Design review of the part built by this model. Coordinates are the model's own, in mm. A direction names the side the tool comes from. Coordinates: 2 decimals unless noted, no trailing zeros. Write each loop counter-clockwise with the first axis right and the second up, starting at its lowest first coordinate (ties: lowest second). Pieces come first, ordered by that corner, then holes. Notation, with made-up numbers: (87, -10.75) - (139, -10.75) arc R28 cw to (139, 19.25) - close; hole circle Ø10 at (-2, 57.25). An arc over 180 degrees is marked (long way). Answer as CSV lines item,"result". Start each with the question number.
Q1. Machinability: for faces 1 (the face through (-11, 10, 6)), 2 (the face through (-23.846, 4.93, -7.509)), which of the approach directions +Z, -Z, +X, -X, +Y, -Y give a long, thin tool a straight path to every point of the face, cutting with its end or side? Answer none if there is none.
Q2. We need section B-B (z = 0). Write out the cut boundary in (x, y), plus the area to 3 significant figures.
Q3. We need section D-D (z = 20). Write out the cut boundary in (x, y), plus the area to 3 significant figures.
Q4. We need section A-A (x = 20). Write out the cut boundary in (y, z), plus the area to 3 significant figures.
Q5. Mouldability with a two-part tool opening along X and no side actions: class faces 3 (the face through (0, 110, 11)), 4 (the face through (-17, 5, 0)), 5 (the face through (-3.2, 59.3, 10)), 6 (the face through (-11.99, 59.3, 0.53)) as pulls with the +X half, pulls with the -X half, needs draft (parallel to the pull), parting line crosses it, or undercut.
Q6. We need section C-C (x = 0). Write out the cut boundary in (y, z).
Q7. For line 1 along Y through (x, z) = (9, 1.5); line 2 along Z through (x, y) = (2.5, 32.5); line 3 along X through (y, z) = (43, 0), list the stretches that pass through material, from the lowest coordinate up. Write a range as [from, to].
Q8. Clearance check with flat-ended pins moving along their axes: pin 1 (10.5 mm diameter, centred on x = 2.5, z = -2, fed in from +Y); pin 2 (5.5 mm diameter, centred on x = -20, z = 0, fed in from +Y); pin 3 (1 mm diameter, centred on y = 21.5, z = 8.5, fed in from +X); pin 4 (5 mm diameter, centred on x = -2.5, y = 76.5, fed in from +Z). State where each tip first meets the part, or that it passes through.
Autodesk Inventor part; units mm, degrees
ref_plane "YZ Plane" through (0, 0, 0) normal (1, 0, 0) x (0, 1, 0)
ref_plane "XZ Plane" through (0, 0, 0) normal (0, 1, 0) x (-1, 0, 0)
ref_plane "XY Plane" through (0, 0, 0) normal (0, 0, 1) x (1, 0, 0)
sketch "Boceto1" plane through (0, 0, 0) normal (0, 1, 0) x (-1, 0, 0)
  circle A0 centre (0, 0) radius 25
  circle A1 centre (20, 0) radius 3
  circle A2 centre (0, 20) radius 3
  circle A3 centre (-20, 0) radius 3
  circle A4 centre (0, -20) radius 3
  dimension "d0" = 50
  dimension "d2" = 6
  dimension "d5" = 360
extrude "Extrusión1" add sketch "Boceto1" along normal blind 10
sketch "Boceto2" plane through (0, 10, 0) normal (0, 1, 0) x (1, 0, 0)
  circle A0 centre (0, 0) radius 12
  circle A1 centre (0, 0) radius 10.5
  dimension "d9" = 24
  dimension "d10" = 21
extrude "Extrusión2" add sketch "Boceto2" along normal blind 100 contours A0 | A1
sketch "Boceto3" plane through (0, 110, 0) normal (0, 1, 0) x (1, 0, 0)
  circle A0 centre (0, 0) radius 12
hole "Agujero1" at (0, 110, 0) direction (0, -1, 0) diameter 21 depth 100
Results list:
1,face 1,"+Y"
1,face 2,"+Y, -Y"
2,outline,"(-25, 0) - (-23, 0) - (-23, 10) - (-25, 10) - close; (-17, 0) - (17, 0) - (17, 10) - (12, 10) - (12, 110) - (10.5, 110) - (10.5, 10) - (-10.5, 10) - (-10.5, 110) - (-12, 110) - (-12, 10) - (-17, 10) - close; (23, 0) - (25, 0) - (25, 10) - (23, 10) - close"
2,area,"680 mm2"
3,outline,"(-15, 0) - (-3, 0) - (-3, 10) - (-15, 10) - close; (3, 0) - (15, 0) - (15, 10) - (3, 10) - close"
3,area,"240 mm2"
4,outline,"(0, -15) - (10, -15) - (10, -3) - (0, -3) - close; (0, 3) - (10, 3) - (10, 15) - (0, 15) - close"
4,area,"240 mm2"
5,face 3,"needs draft"
5,face 4,"undercut"
5,face 5,"undercut"
5,face 6,"parting line crosses it"
6,outline,"(0, -25) - (10, -25) - (10, -23) - (0, -23) - close; (0, -17) - (10, -17) - (10, -12) - (110, -12) - (110, -10.5) - (10, -10.5) - (10, 10.5) - (110, 10.5) - (110, 12) - (10, 12) - (10, 17) - (0, 17) - close; (0, 23) - (10, 23) - (10, 25) - (0, 25) - close"
7,line 1,"y = [0, 10]"
7,line 2,"z = [-11.74, -10.2], [10.2, 11.74]"
7,line 3,"x = [-12, -10.5], [10.5, 12]"
8,pin 1,"stops at y = 10"
8,pin 2,"passes through"
8,pin 3,"stops at x = 8.94"
8,pin 4,"stops at z = 12"
